Part model, mm, in its own coordinate system. Give positions to 0.01 mm unless a question says otherwise; leave off trailing zeros. Order: outer loops, then holes, each group sorted by start corner. A loop starts at its lowest first (then second) coordinate and runs counter-clockwise, first axis right, second up. Notation, with made-up numbers: M 68,48 L 88,48 A26 cw 88,78 Z; hole C -17.5,1 d3. An arc over 180 degrees is marked long. Write each question's results on one line, items separated by ' | '. Start each with the question number.
from build123d import *

# Parameters (mm, degrees)
SKETCH1_R               = 1.75
BOSS_EXTRUDE1_DEPTH     = 1
CUT_EXTRUDE1_DEPTH      = 47.247436748
CUT_EXTRUDE1_DEPTH_BACK = 47.247436748


with BuildPart() as part:
    # Sketch1 → Boss-Extrude1 (new, symmetric)
    with BuildSketch(Plane(origin=(0, 0, 0), x_dir=(1, 0, 0), z_dir=(0, 1, 0))):
        with BuildLine():
            ThreePointArc((-3.074068123, 2.480444551), (-2.35494781, -3.171233327), (3.263278519, -2.225648963))
            ThreePointArc((3.263278519, -2.225648963), (19.240732221, 6.066624624), (34.966250056, -2.694021293))
            ThreePointArc((34.966250056, -2.694021293), (42.169032262, -4.007012426), (42.959429057, 3.271674965))
            ThreePointArc((42.959429057, 3.271674965), (19.757716522, 13.637194671), (-3.074068123, 2.480444551))
        make_face()
        with Locations(Location((0, 0, 0), (0, 0, 270))):
            Circle(SKETCH1_R, mode=Mode.SUBTRACT)
        with Locations(Location((39.178405, 0, 0), (0, 0, 270))):
            Circle(SKETCH1_R, mode=Mode.SUBTRACT)
    extrude(amount=BOSS_EXTRUDE1_DEPTH, both=True)

    # Sketch2 → Cut-Extrude1 (cut, two sides: drawn at the far end of the back side and taken through both)
    with BuildSketch(Plane(origin=(0, 0, 0), x_dir=(1, 0, 0), z_dir=(0, 1, 0)).offset(-CUT_EXTRUDE1_DEPTH_BACK)):
        Polygon((36.17646787, -5.383387255), (31.918373047, 5.155767261), (14.230811062, -1.990471652), (18.488905885, -12.529626168), align=None)
    extrude(amount=CUT_EXTRUDE1_DEPTH + CUT_EXTRUDE1_DEPTH_BACK, mode=Mode.SUBTRACT)


solid = part.part
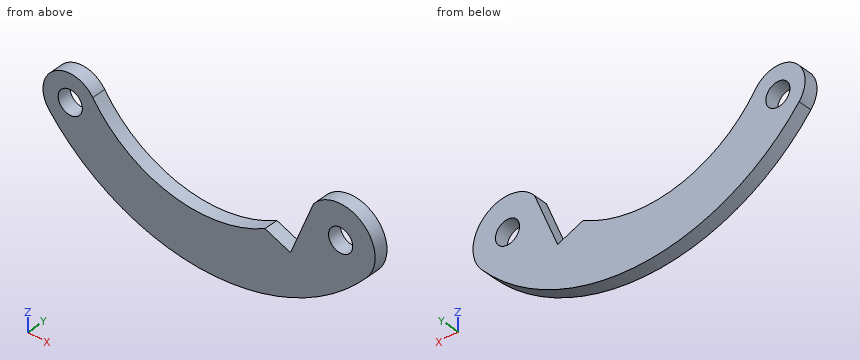
(1) Saw through at A-A on x = 1. Give the cut face in (y, z).
(2) Probe L1, parallel to X at y = 0.2, z = 1; L2, parallel to X at y = 0.15, z = 0; L3, parallel to X at y = 0.9, z = -4.5. List the from-to ranges inside material, lowest first.
(3) Saw through at C-C on y = 0.2. Give the cut face in (x, z).
(4) Saw through at D-D on z = -7.75. Give the cut face in (x, y).
(5) Saw through at B-B on z = 0. Give the cut face in (x, y), plus the area to 3 significant figures.
Taken from the geometry:
1) outline: M -1,-6.63 L 1,-6.63 L 1,-1.44 L -1,-1.44 Z; M -1,1.44 L 1,1.44 L 1,3.82 L -1,3.82 Z
2) L1: x = -3.82 to -1.44, 1.44 to 4.17, 34.41 to 37.74, 40.61 to 44.08 | L2: x = -3.95 to -1.75, 1.75 to 5.04, 34 to 37.43, 40.93 to 44.18 | L3: x = -1.29 to 11.4, 26.52 to 30.3, 32.18 to 41.84
3) outline: M -3.07,-2.48 A30 ccw 42.96,-3.27 A5 ccw long 35.25,3.1 L 31.92,-5.16 L 28.22,-3.66 A19 cw 3.26,2.23 A3.95 ccw long Z; hole C 0,0 d3.5; hole C 39.18,0 d3.5
4) outline: M 2.42,-1 L 38.13,-1 L 38.13,1 L 2.42,1 Z
5) outline: M -3.95,-1 L -1.75,-1 L -1.75,1 L -3.95,1 Z; M 1.75,-1 L 5.04,-1 L 5.04,1 L 1.75,1 Z; M 34,-1 L 37.43,-1 L 37.43,1 L 34,1 Z; M 40.93,-1 L 44.18,-1 L 44.18,1 L 40.93,1 Z | area: 24.3 mm²
